Design review of the part built by this model. Coordinates are the model's own, in mm. A direction names the side the tool comes from. Round coordinates to 2 decimals unless told otherwise and drop trailing zeros. Loops run counter-clockwise (first coordinate to the right, second up) from the corner with the lowest first, then second, coordinate; pieces in that order, holes last. Notation, with made-up numbers: M 55.5,-7.5 L 73.5,-7.5 A19 ccw 73.5,20.5 Z; hole C 12.25,-39.75 d4. An arc over 180 degrees is marked long. Answer as CSV lines item,"result". Start each with the question number.
from build123d import *

# Parameters (mm, degrees)
F0_W     = 1500
F0_H     = 1000
F1_DEPTH = 750
F2_W     = 1250
F2_H     = 750
F3_DEPTH = 350
F4_W     = 250
F4_H     = 750
F5_DEPTH = 150


with BuildPart() as f1:
    # F0 (on Top) → F1 (new body)
    with BuildSketch(Plane.XY):
        Rectangle(F0_W, F0_H)
    extrude(amount=F1_DEPTH)

    # F2 (on face) → F3 (cut)
    with BuildSketch(Plane.XY.offset(750)):
        with Locations((-125, -125)):
            Rectangle(F2_W, F2_H)
    extrude(amount=-F3_DEPTH, mode=Mode.SUBTRACT)

    # F4 (on face) → F5 (cut)
    with BuildSketch(Plane.XY.offset(750)):
        with Locations((625, -125)):
            Rectangle(F4_W, F4_H)
    extrude(amount=-F5_DEPTH, mode=Mode.SUBTRACT)


solid = f1.part
Item 1: Insertion check: pin 1 Ø10 at (x, y) = (120.5, 26.5) entering from +Z; pin 2 Ø2 at (x, y) = (-132, -266.5) entering from -Z. Each pin has a flat end and moves straight along its axis. Give the tip position at first contact, or say it passes through.
Item 2: Consider section B-B, the plane y = -281.5. Write out the cut boundary in (x, z), then the cut area to 3 significant figures.
Item 3: Consider section C-C, the plane z = 664. Write out the cut boundary in (x, y), then the cut area to 3 significant figures.
Item 4: To check wall thickness, follow line 1 (Y direction, x = -449, z = 531); line 2 (Z direction, x = -145.5, y = 87); line 3 (X direction, y = -56.5, z = 524.5). State the ranges of each line that lie inside material, in increasing order.
Item 5: Tool access review of faces 1 (the face through (623, -120, 600)), 2 (the face through (500, -130, 501)), 3 (the face through (-10, -500, 229)): name each direction out of +Z, -Z, +X, -X, +Y, -Y from which nothing blocks a thin tool from reaching the whole face with its end or side.
Item 6: Consider section A-A, the plane x = -540.5. Write out the cut boundary in (y, z), then the cut area to 4 significant figures.
Found:
1,pin 1,"stops at z = 400"
1,pin 2,"stops at z = 0"
2,outline,"M -750,0 L 750,0 L 750,600 L 500,600 L 500,400 L -750,400 Z"
2,area,"650,000 mm^2"
3,outline,"M -750,250 L 750,250 L 750,500 L -750,500 Z"
3,area,"375,000 mm^2"
4,line 1,"y = 250 to 500"
4,line 2,"z = 0 to 400"
4,line 3,"x = 500 to 750"
5,face 1,"+Z, +X, -X, -Y"
5,face 2,"+Z, -X, -Y"
5,face 3,"+Z, -Z, +X, -X, -Y"
6,outline,"M -500,0 L 500,0 L 500,750 L 250,750 L 250,400 L -500,400 Z"
6,area,"487,500 mm^2"
